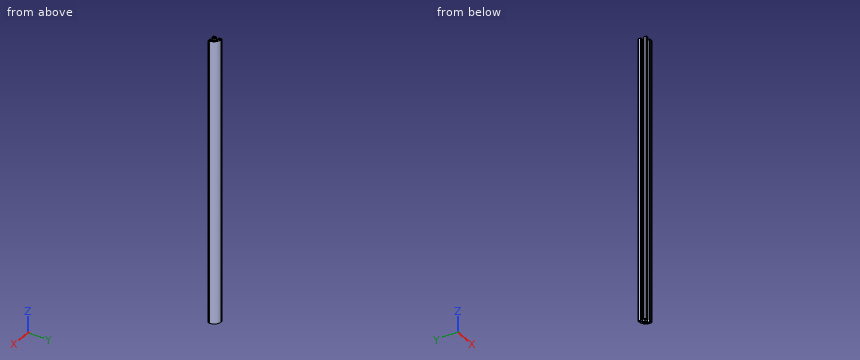
from build123d import *

# Parameters (mm, degrees)
SKETCH_1_R      = 3.4
EXTRUDE_1_DEPTH = 1000


with BuildPart() as part:
    # Эскиз1 → Бобышка-Вытянуть1 (new body)
    with BuildSketch(Plane.XY):
        with BuildLine():
            Line((-15, -5.5), (-15, -8.25))
            Line((-15, -8.25), (-15, -13))
            ThreePointArc((-15, -13), (-14.414213562, -14.414213562), (-13, -15))
            Line((-13, -15), (-8.25, -15))
            Line((-8.25, -15), (-5.5, -15))
            ThreePointArc((-5.5, -15), (-5.287867966, -14.912132034), (-5.2, -14.7))
            Line((-5.2, -14.7), (-5.2, -14))
            Line((-5.2, -14), (-4.4, -14))
            ThreePointArc((-4.4, -14), (-4.187867966, -13.912132034), (-4.1, -13.7))
            Line((-4.1, -13.7), (-4.1, -13.1))
            ThreePointArc((-4.1, -13.1), (-4.187867966, -12.887867966), (-4.4, -12.8))
            Line((-4.4, -12.8), (-7.95, -12.8))
            ThreePointArc((-7.95, -12.8), (-8.162132034, -12.712132034), (-8.25, -12.5))
            Line((-8.25, -12.5), (-8.25, -9.8))
            Line((-8.25, -9.8), (-4.25, -5.8))
            Line((-4.25, -5.8), (4.25, -5.8))
            Line((4.25, -5.8), (8.25, -9.8))
            Line((8.25, -9.8), (8.25, -12.5))
            ThreePointArc((8.25, -12.5), (8.162132034, -12.712132034), (7.95, -12.8))
            Line((7.95, -12.8), (4.4, -12.8))
            ThreePointArc((4.4, -12.8), (4.187867966, -12.887867966), (4.1, -13.1))
            Line((4.1, -13.1), (4.1, -13.7))
            ThreePointArc((4.1, -13.7), (4.187867966, -13.912132034), (4.4, -14))
            Line((4.4, -14), (5.2, -14))
            Line((5.2, -14), (5.2, -14.7))
            ThreePointArc((5.2, -14.7), (5.287867966, -14.912132034), (5.5, -15))
            Line((5.5, -15), (8.25, -15))
            Line((8.25, -15), (13, -15))
            ThreePointArc((13, -15), (14.414213562, -14.414213562), (15, -13))
            Line((15, -13), (15, -10))
            ThreePointArc((15, -10), (7.67766953, 7.67766953), (-10, 15))
            Line((-10, 15), (-13, 15))
            ThreePointArc((-13, 15), (-14.414213562, 14.414213562), (-15, 13))
            Line((-15, 13), (-15, 8.25))
            Line((-15, 8.25), (-15, 5.5))
            ThreePointArc((-15, 5.5), (-14.912132034, 5.287867966), (-14.7, 5.2))
            Line((-14.7, 5.2), (-14, 5.2))
            Line((-14, 5.2), (-14, 4.4))
            ThreePointArc((-14, 4.4), (-13.912132034, 4.187867966), (-13.7, 4.1))
            Line((-13.7, 4.1), (-13.1, 4.1))
            ThreePointArc((-13.1, 4.1), (-12.887867966, 4.187867966), (-12.8, 4.4))
            Line((-12.8, 4.4), (-12.8, 7.95))
            ThreePointArc((-12.8, 7.95), (-12.712132034, 8.162132034), (-12.5, 8.25))
            Line((-12.5, 8.25), (-9.8, 8.25))
            Line((-9.8, 8.25), (-5.8, 4.25))
            Line((-5.8, 4.25), (-5.8, -4.25))
            Line((-5.8, -4.25), (-9.8, -8.25))
            Line((-9.8, -8.25), (-12.5, -8.25))
            ThreePointArc((-12.5, -8.25), (-12.712132034, -8.162132034), (-12.8, -7.95))
            Line((-12.8, -7.95), (-12.8, -4.4))
            ThreePointArc((-12.8, -4.4), (-12.887867966, -4.187867966), (-13.1, -4.1))
            Line((-13.1, -4.1), (-13.7, -4.1))
            ThreePointArc((-13.7, -4.1), (-13.912132034, -4.187867966), (-14, -4.4))
            Line((-14, -4.4), (-14, -5.2))
            Line((-14, -5.2), (-14.7, -5.2))
            ThreePointArc((-14.7, -5.2), (-14.912132034, -5.287867966), (-15, -5.5))
        make_face()
        with BuildLine():
            ThreePointArc((-13.15, -10.35), (-13.003553391, -9.996446609), (-12.65, -9.85))
            Line((-12.65, -9.85), (-10.35, -9.85))
            ThreePointArc((-10.35, -9.85), (-9.996446609, -9.996446609), (-9.85, -10.35))
            Line((-9.85, -10.35), (-9.85, -12.65))
            ThreePointArc((-9.85, -12.65), (-9.996446609, -13.003553391), (-10.35, -13.15))
            Line((-10.35, -13.15), (-12.65, -13.15))
            ThreePointArc((-12.65, -13.15), (-13.003553391, -13.003553391), (-13.15, -12.65))
            Line((-13.15, -12.65), (-13.15, -10.35))
        make_face(mode=Mode.SUBTRACT)
        Circle(SKETCH_1_R, mode=Mode.SUBTRACT)
        with BuildLine():
            Line((13, -10), (13, -12.5))
            ThreePointArc((13, -12.5), (12.853553391, -12.853553391), (12.5, -13))
            Line((12.5, -13), (10.75, -13))
            ThreePointArc((10.75, -13), (10.396446609, -12.853553391), (10.25, -12.5))
            Line((10.25, -12.5), (10.25, -8.895836944))
            ThreePointArc((10.25, -8.895836944), (10.211939766, -8.704495228), (10.103553391, -8.542283553))
            Line((10.103553391, -8.542283553), (5.846446609, -4.285176772))
            ThreePointArc((5.846446609, -4.285176772), (5.738060234, -4.122965098), (5.7, -3.931623382))
            Line((5.7, -3.931623382), (5.7, 3.854163056))
            ThreePointArc((5.7, 3.854163056), (5.738060234, 4.045504772), (5.846446609, 4.207716447))
            Line((5.846446609, 4.207716447), (6.685973486, 5.047243323))
            ThreePointArc((6.685973486, 5.047243323), (7.057970063, 5.193349665), (7.418183029, 5.020216375))
            ThreePointArc((7.418183029, 5.020216375), (11.559431923, -1.988077936), (13, -10))
        make_face(mode=Mode.SUBTRACT)
        with BuildLine():
            Line((-13, 10.75), (-13, 12.5))
            ThreePointArc((-13, 12.5), (-12.853553391, 12.853553391), (-12.5, 13))
            Line((-12.5, 13), (-10, 13))
            ThreePointArc((-10, 13), (-1.988077936, 11.559431923), (5.020216375, 7.418183029))
            ThreePointArc((5.020216375, 7.418183029), (5.193349665, 7.057970063), (5.047243323, 6.685973486))
            Line((5.047243323, 6.685973486), (4.207716447, 5.846446609))
            ThreePointArc((4.207716447, 5.846446609), (4.045504772, 5.738060234), (3.854163056, 5.7))
            Line((3.854163056, 5.7), (-3.931623382, 5.7))
            ThreePointArc((-3.931623382, 5.7), (-4.122965098, 5.738060234), (-4.285176772, 5.846446609))
            Line((-4.285176772, 5.846446609), (-8.542283553, 10.103553391))
            ThreePointArc((-8.542283553, 10.103553391), (-8.704495228, 10.211939766), (-8.895836944, 10.25))
            Line((-8.895836944, 10.25), (-12.5, 10.25))
            ThreePointArc((-12.5, 10.25), (-12.853553391, 10.396446609), (-13, 10.75))
        make_face(mode=Mode.SUBTRACT)
    extrude(amount=EXTRUDE_1_DEPTH)


solid = part.part
For this review, take the finished solid that the model builds, in its own axes (mm). Give positions to 0.01 mm unless a question says otherwise; leave off trailing zeros. Put each result on its own line as item: value. Start each with the question number.
(1) Wall thickness on L1, parallel to X at y = -12.75, z = 257.5; L2, parallel to Y at x = 0, z = 759; L3, parallel to Y at x = -9.75, z = 612: over which ranges is each line inside the solid? List them lowest first.
(2) Add section A-A, the plane z = 668. Give the number of separate pieces and of enclosed holes in the cut face, then the cut area to 3 significant figures.
(3) For pin 1 (0.8 mm diameter, centred on y = -14, z = 387, fed in from -X); pin 2 (0.9 mm diameter, centred on y = 5, z = 513, fed in from -X); pin 3 (10 mm diameter, centred on x = -1, z = 715.5, fed in from +Y), all flat-tipped, find the tip position at first contact; note any pin that passes through.
Result:
1. L1: x = -15 to -13.14, -9.86 to -8.12, 8.12 to 10.32, 12.93 to 15
1. L2: y = -5.8 to -3.4, 3.4 to 5.7, 10.71 to 12.91
1. L3: y = -15 to -8.2, 8.2 to 10.25, 13 to 15
2. separate pieces: 1
2. enclosed holes: 4
2. area: 327 mm^2
3. pin 1: stops at x = -14.91
3. pin 2: stops at x = -15
3. pin 3: stops at y = 14.68
